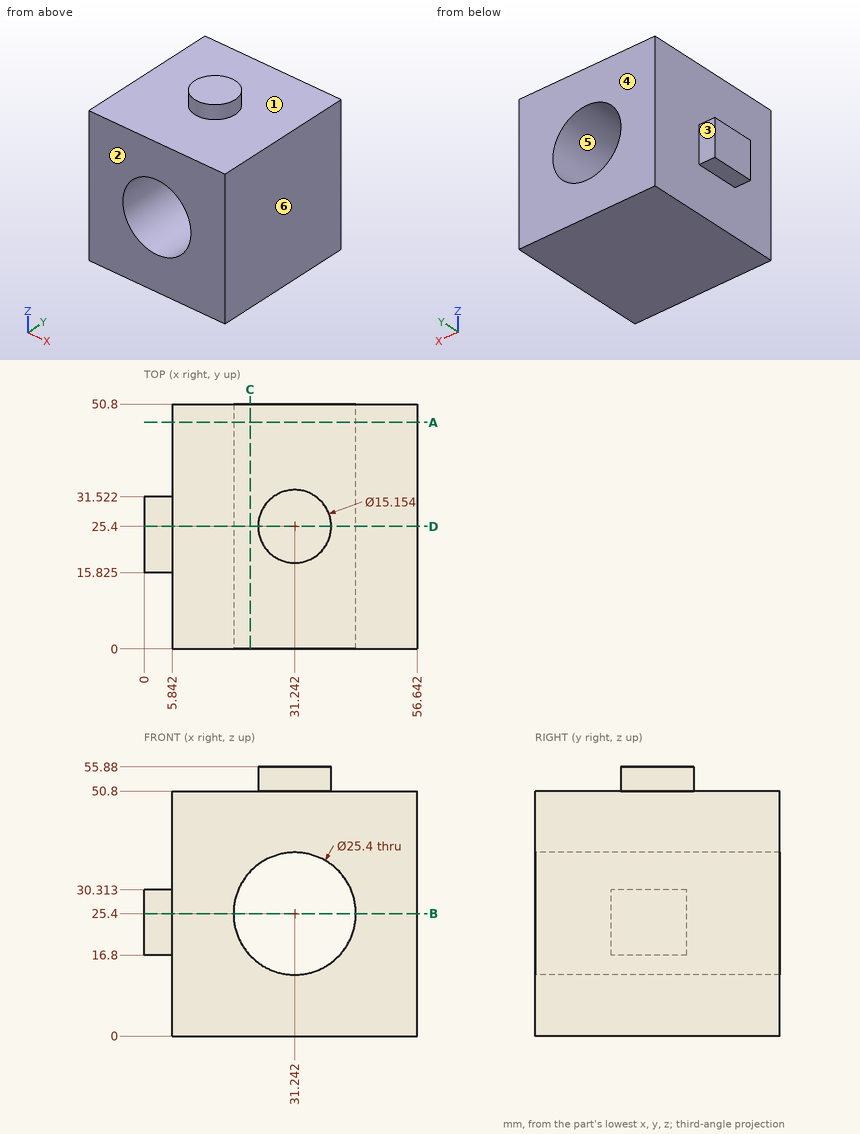
The figure shows three views and two pictorial views of one solid part (mm, origin at its lowest corner). Answer the questions. A direction names the side the tool comes from. Round coordinates to 2 decimals unless told otherwise and drop trailing zeros. Loops run counter-clockwise (first coordinate to the right, second up) from the corner with the lowest first, then second, coordinate; pieces in that order, holes last. Notation, with made-up numbers: (3, -1.5) - (9, -1.5) arc R11 ccw to (9, 11.5) - close; hole circle Ø11 at (29, -2.5). An arc over 180 degrees is marked (long way). One line per question, with ' | ' between items. Start each with the question number.
Q1. For a pull along X with two mould halves and no side action, classify the marked faces 4, 5 and 6 as +X half, -X half, draft (parallel to the pull), parting line (faces both ways), or undercut.
Q2. For the marked faces 1, 2 and 3, determine the directions among +Z, -Z, +X, -X, +Y, -Y from which every point of the face is accessible in a straight line to the end or side of a thin tool.
Q3. Section D-D on y = 25.4 is taken. Give the vertices of the cut face in (x, z) (1 decimal).
Q4. Section B-B on z = 25.4 is taken. Give the vertices of the cut face in (x, y) (1 decimal).
Q5. Section A-A on y = 47 is taken. Give the vertices of the cut face in (x, z).
Q6. Section C-C on x = 22 is taken. Give the vertices of the cut face in (y, z).
Q7. Find the intervals of material crossed by L1, parallel to X at y = 14, z = 25 (1 decimal); L2, parallel to X at y = 20, z = 25 (1 decimal); L3, parallel to X at y = 43.5, z = 46, in increasing order.
Q8. Flat-ended cylindrical pins translate along their axes: pin 1 (4.5 mm diameter, centred on x = 3, z = 21, fed in from +Y); pin 2 (15 mm diameter, centred on y = 23, z = 32, fed in from -X); pin 3 (5 mm diameter, centred on x = 39, y = 37.5, fed in from +Z); pin 4 (4.5 mm diameter, centred on x = 3, y = 25, fed in from +Z). Find the tip coordinate at first contact, or state that the pin passes through.
Established:
1) face 4: draft | face 5: undercut | face 6: +X half
2) face 1: +Z | face 2: +Z, -Z, +X, -X, -Y | face 3: +Z, -Z, -X, +Y
3) outline: (0, 16.8) - (5.8, 16.8) - (5.8, 0) - (56.6, 0) - (56.6, 50.8) - (38.8, 50.8) - (38.8, 55.9) - (23.7, 55.9) - (23.7, 50.8) - (5.8, 50.8) - (5.8, 30.3) - (0, 30.3) - close; hole circle Ø25.4 at (31.2, 25.4)
4) outline: (0, 15.8) - (5.8, 15.8) - (5.8, 0) - (18.5, 0) - (18.5, 50.8) - (5.8, 50.8) - (5.8, 31.5) - (0, 31.5) - close; (43.9, 0) - (56.6, 0) - (56.6, 50.8) - (43.9, 50.8) - close
5) outline: (5.84, 0) - (56.64, 0) - (56.64, 50.8) - (5.84, 50.8) - close; hole circle Ø25.4 at (31.24, 25.4)
6) outline: (0, 0) - (50.8, 0) - (50.8, 16.69) - (0, 16.69) - close; (0, 34.11) - (50.8, 34.11) - (50.8, 50.8) - (0, 50.8) - close
7) L1: 5.8 to 18.5, 43.9 to 56.6 | L2: 0 to 18.5, 43.9 to 56.6 | L3: 5.84 to 56.64
8) pin 1: y = 31.52 | pin 2: x = 0 | pin 3: z = 50.8 | pin 4: z = 30.31
